from build123d import *

# Parameters (mm, degrees)
SKETCH1_R           = 12.192
BOSS_EXTRUDE1_DEPTH = 30.48
SKETCH2_R           = 3.175
BOSS_EXTRUDE2_DEPTH = 1.778
SKETCH3_R           = 1.016
BOSS_EXTRUDE3_DEPTH = 14.224
FILLET1_R           = 1.016
FILLET2_R           = 1.016


with BuildPart() as part:
    # Sketch1 → Boss-Extrude1 (new body)
    with BuildSketch(Plane(origin=(0, 0, 0), x_dir=(1, 0, 0), z_dir=(0, 1, 0))):
        with Locations(Location((0, 0, 0), (0, 0, 90))):
            Circle(SKETCH1_R)
    extrude(amount=BOSS_EXTRUDE1_DEPTH)

    # Sketch2 → Boss-Extrude2 (add)
    with BuildSketch(Plane(origin=(0, 30.48, 0), x_dir=(1, 0, 0), z_dir=(0, 1, 0))):
        with Locations(Location((0, 0, 0), (0, 0, 270))):
            Circle(SKETCH2_R)
    extrude(amount=BOSS_EXTRUDE2_DEPTH)

    # Sketch3 → Boss-Extrude3 (add)
    with BuildSketch(Plane(origin=(0, 32.258, 0), x_dir=(1, 0, 0), z_dir=(0, 1, 0))):
        with Locations(Location((0, 0, 0), (0, 0, 270))):
            Circle(SKETCH3_R)
    extrude(amount=BOSS_EXTRUDE3_DEPTH)

    # Fillet1
    fillet1_edges = [part.edges().sort_by_distance(p)[0] for p in [
        (0, 46.482, -1.016),
    ]]
    fillet(fillet1_edges, radius=FILLET1_R)

    # Fillet2
    fillet2_edges = [part.edges().sort_by_distance(p)[0] for p in [
        (0, 30.48, 12.192),
    ]]
    fillet(fillet2_edges, radius=FILLET2_R)


solid = part.part
Can you work these out from the model? Positions are in its coordinate system, mm. A direction names the side the tool comes from. Coordinates: 2 decimals unless noted, no trailing zeros. Order: outer loops, then holes, each group sorted by start corner. A loop starts at its lowest first (then second) coordinate and runs counter-clockwise, first axis right, second up. Notation, with made-up numbers: M 40.25,39 L 76.25,39 A33 cw 76.25,72 Z; hole C 37,89 d10. An arc over 180 degrees is marked long. Answer as CSV lines item,"result".
(1) Suppose I cut it at C-C on y = 42. Please give me the cut outline in (x, z).
Geometry check:
outline,"C 0,0 d2.03"
(2) On a 3-axis mill with a long thin cutter (end or side, diameter ignored), from which of +Z, -Z, +X, -X, +Y, -Y can I reach the whole of each face in a straight line? I mean faces 1 (the cylindrical face through (-10.28, 14.526, -6.554)), 2 (the cylindrical face through (-1.93, 31.36, -2.52)). Say none if no direction works.
Geometry check:
face 1,"+Y, -Y"
face 2,"+Y"
(3) Suppose I cut it at A-A on z = 0. Please give me the cut outline in (x, y) (3 decimals).
Geometry check:
outline,"M -12.192,0 L 12.192,0 L 12.192,29.464 A1.016 ccw 11.176,30.48 L 3.175,30.48 L 3.175,32.258 L 1.016,32.258 L 1.016,45.466 A1.016 ccw -1.016,45.466 L -1.016,32.258 L -3.175,32.258 L -3.175,30.48 L -11.176,30.48 A1.016 ccw -12.192,29.464 Z"
(4) I'm going to push flat-ended pins straight in: pin 1 (4 mm diameter, centred on x = -6.5, y = 8.5, fed in from -Z); pin 2 (8 mm diameter, centred on x = 6.5, y = 32, fed in from +Z); pin 3 (1 mm diameter, centred on y = 9, z = 9, fed in from -X). Where does each tip first touch, or does it pass through?
Geometry check:
pin 1,"z = -11.33"
pin 2,"z = 11.73"
pin 3,"x = -8.74"
(5) Suppose I cut it at B-B on x = 0. Please give me the cut outline in (y, z) (3 decimals).
Geometry check:
outline,"M 0,-12.192 L 29.464,-12.192 A1.016 ccw 30.48,-11.176 L 30.48,-3.175 L 32.258,-3.175 L 32.258,-1.016 L 45.466,-1.016 A1.016 ccw 45.466,1.016 L 32.258,1.016 L 32.258,3.175 L 30.48,3.175 L 30.48,11.176 A1.016 ccw 29.464,12.192 L 0,12.192 Z"
(6) Please list where these lines run through material, in increasing order: L1, parallel to Y at x = 6.5, z = 5.25; L2, parallel to X at y = 12, z = -0.25; L3, parallel to Z at x = -5, y = 26.5.
Geometry check:
L1,"0 to 30.48"
L2,"-12.19 to 12.19"
L3,"-11.12 to 11.12"
